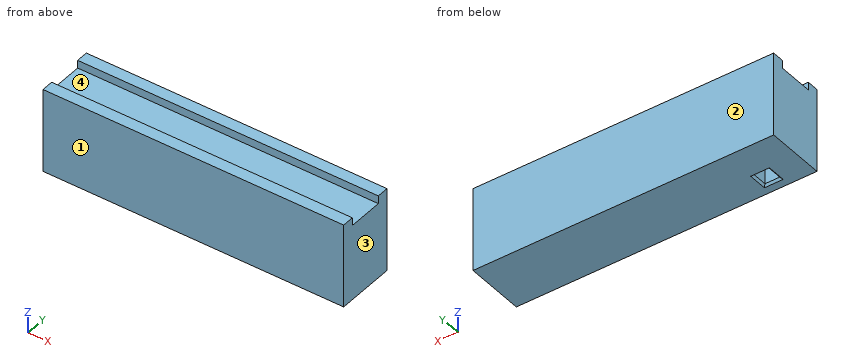
from build123d import *

# Parameters (mm, degrees)
PAD001_DEPTH    = 30.48
SKETCH003_W     = 1.5
SKETCH003_H     = 1.5
POCKET_DEPTH    = 7.5
CHAMFER008_SIZE = 0.2


with BuildPart() as part:
    # Sketch001 → Pad001 (new body)
    with BuildSketch(Plane.YZ.offset(-3.51)):
        Polygon((0, 8.5), (1.2, 8.5), (1.2, 7.7), (4.8, 7.7), (4.8, 8.5), (6, 8.5), (6, 0), (0, 0), align=None)
    extrude(amount=PAD001_DEPTH)

    # Sketch003 → Pocket (cut)
    with BuildSketch(Plane(origin=(-3.51, 0, 0), x_dir=(0, 1, 0), z_dir=(0, 0, -1))):
        with Locations((1.73, 3.81)):
            Rectangle(SKETCH003_W, SKETCH003_H)
    extrude(amount=-POCKET_DEPTH, mode=Mode.SUBTRACT)

    # Chamfer008
    chamfer008_edges = [part.edges().sort_by_distance(p)[0] for p in [
        (-0.45, 1.73, 0),
        (0.3, 2.48, 0),
        (1.05, 1.73, 0),
        (0.3, 0.98, 0),
    ]]
    chamfer(chamfer008_edges, length=CHAMFER008_SIZE)


solid = part.part
Verification items for the finished model (mm, model axes). Face numbers are marked on the shaded views. Round coordinates to 2 decimals unless told otherwise and drop trailing zeros. Order: outer loops, then holes, each group sorted by start corner. A loop starts at its lowest first (then second) coordinate and runs counter-clockwise, first axis right, second up.
1. Thickness scan on L1, parallel to X at y = 2.1, z = 2; L2, parallel to Y at x = 21, z = 8; L3, parallel to Y at x = 0, z = 4.25. Record the ranges inside material, lowest first.
Final values:
L1: x = -3.51 to -0.45, 1.05 to 26.97
L2: y = 0 to 1.2, 4.8 to 6
L3: y = 0 to 0.98, 2.48 to 6
2. Go/stop test with a flat-tipped pin: P1, Ø2, axis at x = 17.5, y = 2.5, coming from the +Z side. Record where the tip stops, or that it passes through.
Final values:
P1: stops at z = 7.7
3. Release check for a two-part mould opening along Y. For the marked faces 1, 2, 3 and 4 record: +Y half, -Y half, draft (parallel to the pull), parting line (faces both ways), or undercut.
Final values:
face 1: -Y half
face 2: +Y half
face 3: draft
face 4: undercut
4. Section check A-A on x = 7.5. Record the cut outline in (y, z).
Final values:
outline: (0, 0) - (6, 0) - (6, 8.5) - (4.8, 8.5) - (4.8, 7.7) - (1.2, 7.7) - (1.2, 8.5) - (0, 8.5) - close
